Source: CAD feature listing. Evaluate the final solid. Frame: model axes, mm. A direction names the side the tool comes from. Give positions to 0.01 mm unless a question says otherwise; leave off trailing zeros. Write each loop counter-clockwise with the first axis right and the second up, starting at its lowest first coordinate (ties: lowest second). Pieces come first, ordered by that corner, then holes. Notation, with made-up numbers: (53.5, -14) -> (75.5, -14) arc R9 cw to (75.5, -7) -> close; hole circle Ø5 at (-4, 65.25). An arc over 180 degrees is marked (long way). Write item = value, one per line.
Autodesk Inventor part; units mm, degrees
ref_plane "YZ Plane" through (0, 0, 0) normal (1, 0, 0) x (0, 1, 0)
ref_plane "XZ Plane" through (0, 0, 0) normal (0, 1, 0) x (-1, 0, 0)
ref_plane "XY Plane" through (0, 0, 0) normal (0, 0, 1) x (1, 0, 0)
sketch "Sketch1" plane through (0, 0, 0) normal (0, 0, 1) x (1, 0, 0)
  line L0 (-57.5, 17.5) -> (57.5, 17.5)
  line L1 (57.5, 17.5) -> (57.5, -17.5)
  line L2 (57.5, -17.5) -> (-57.5, -17.5)
  line L3 (-57.5, -17.5) -> (-57.5, 17.5)
  line L4 (-57.5, 17.5) -> (57.5, -17.5) construction
  line L5 (57.5, 17.5) -> (-57.5, -17.5) construction
  point P0 (0, 0)
  dimension "d0" = 115
  dimension "d1" = 35
extrude "Extrusion1" add sketch "Sketch1" along normal blind 5
sketch "Sketch2" plane through (0, 0, 5) normal (0, 0, 1) x (1, 0, 0)
  line L0 (57.5, 17.5) -> (-57.5, 17.5)
  line L1 (-33.5, -17.5) -> (33.5, -17.5)
  line L2 (33.5, -17.5) -> (33.5, 17.5)
  line L3 (33.5, 17.5) -> (-33.5, 17.5)
  line L4 (-33.5, 17.5) -> (-33.5, -17.5)
  line L5 (-33.5, -17.5) -> (33.5, 17.5) construction
  line L6 (33.5, -17.5) -> (-33.5, 17.5) construction
  point P0 (0, 0)
  dimension "d10" = 67
extrude "Extrusion2" add sketch "Sketch2" along normal blind 60
shell "Shell1" thickness 3 removed faces 1 at (11.1667, -5.8333, 65)
sketch "Sketch3" plane through (0, 0, 0) normal (0, 0, -1) x (-1, 0, 0)
  circle A0 centre (0, 0) radius 5
  circle A1 centre (21, 0) radius 5
  circle A2 centre (-21, 0) radius 5
  circle A3 centre (48.5, 0) radius 4.25
  circle A4 centre (-48.5, 0) radius 4.25
  line L0 (-57.5, -17.5) -> (-57.5, 17.5)
  line L1 (57.5, 17.5) -> (57.5, -17.5)
  dimension "d14" = 10
  dimension "d15" = 10
  dimension "d16" = 10
  dimension "d17" = 21
  dimension "d18" = 21
  dimension "d19" = 8.5
  dimension "d20" = 8.5
  dimension "d21" = 97
  dimension "d22" = 9
  dimension "d23" = 9
extrude "Extrusion3" cut sketch "Sketch3" against normal through all
sketch "Sketch4" plane through (-57.5, -17.5, 0) normal (0, -1, 0) x (1, 0, 0)
  point P0 (57.5, 0)
sketch "Sketch5" plane through (-57.5, -17.5, 0) normal (0, -1, 0) x (1, 0, 0)
  circle A0 centre (57.5, 59) radius 5
  line L0 (24, 65) -> (91, 65)
  point P0 (57.5, 0)
  dimension "d26" = 10
  dimension "d27" = 6
extrude "Extrusion4" cut sketch "Sketch5" against normal blind 3
properties part number "BASE"
(1) Access query for faces 5 (the face through (-43, 0, 5)), 6 (the face through (33.5, 0, 35)), 7 (the face through (57.5, 0, 2)), 8 (the face through (-30.5, 0, 34)), 9 (the face through (-3, -15, 65)). Directions: +Z, -Z, +X, -X, +Y, -Y. A direction counts if a zero-diameter tool reaches every point of the face in a straight line with its end or side. Return the directions, or none.
Values follow:
face_5 = +Z, -X, +Y, -Y
face_6 = +Z, +X, +Y, -Y
face_7 = +Z, -Z, +X, +Y, -Y
face_8 = +Z
face_9 = +Z, +X, -X, +Y, -Y
(2) First-contact query: pin 1 (9 mm diameter, centred on x = 0, y = 0, fed in from +Z); pin 2 (1.5 mm diameter, centred on y = -10, z = 19, fed in from -X); pin 3 (10 mm diameter, centred on y = 6, z = 47.5, fed in from +X); pin 4 (11 mm diameter, centred on x = -48.5, y = 0, fed in from +Z). Flat tips, straight axial feed; report the tip coordinate or a pass-through.
Values follow:
pin_1 = through
pin_2 = -33.5
pin_3 = 33.5
pin_4 = 5
(3) Section query A-A (x = 0). Return loops of the section in (y, z), plus the area to 3 significant figures.
Values follow:
outline = (-17.5, 0) -> (-5, 0) -> (-5, 3) -> (-14.5, 3) -> (-14.5, 54) -> (-17.5, 54) -> close; (-17.5, 64) -> (-14.5, 64) -> (-14.5, 65) -> (-17.5, 65) -> close; (5, 0) -> (17.5, 0) -> (17.5, 65) -> (14.5, 65) -> (14.5, 3) -> (5, 3) -> close
area = 417 mm2
(4) Material intervals for line 1 (X direction, y = 0, z = 48); line 2 (Y direction, x = 18.5, z = 29.5); line 3 (Y direction, x = 0, z = 2.3), sorted ascending.
Values follow:
line_1 = -33.5 to -30.5, 30.5 to 33.5
line_2 = -17.5 to -14.5, 14.5 to 17.5
line_3 = -17.5 to -5, 5 to 17.5
(5) Pull-direction query (X, two-part tool) for faces 1 (the face through (-0.651, -16.021, 63.957)), 2 (the face through (43, 0, 5)), 3 (the face through (0, -14.5, 34)), 4 (the face through (-57.5, 0, 2)); classes: pulls with the +X half, pulls with the -X half, needs draft (parallel to the pull), parting line crosses it, or undercut.
Values follow:
face_1 = undercut
face_2 = needs draft
face_3 = undercut
face_4 = pulls with the -X half
(6) Section query C-C (y = 0). Give the number of separate pieces and of enclosed holes in the cut face, plus the area to 3 significant figures.
Values follow:
separate_pieces = 6
enclosed_holes = 0
area = 638 mm2
(7) Section query B-B (x = -21). Return loops of the section in (y, z).
Values follow:
outline = (-17.5, 0) -> (-5, 0) -> (-5, 3) -> (-14.5, 3) -> (-14.5, 65) -> (-17.5, 65) -> close; (5, 0) -> (17.5, 0) -> (17.5, 65) -> (14.5, 65) -> (14.5, 3) -> (5, 3) -> close
(8) Section query D-D (z = 29). Return loops of the section in (x, y), plus the area to 3 significant figures.
Values follow:
outline = (-33.5, -17.5) -> (33.5, -17.5) -> (33.5, 17.5) -> (-33.5, 17.5) -> close; hole (-30.5, -14.5) -> (30.5, -14.5) -> (30.5, 14.5) -> (-30.5, 14.5) -> close
area = 576 mm2
